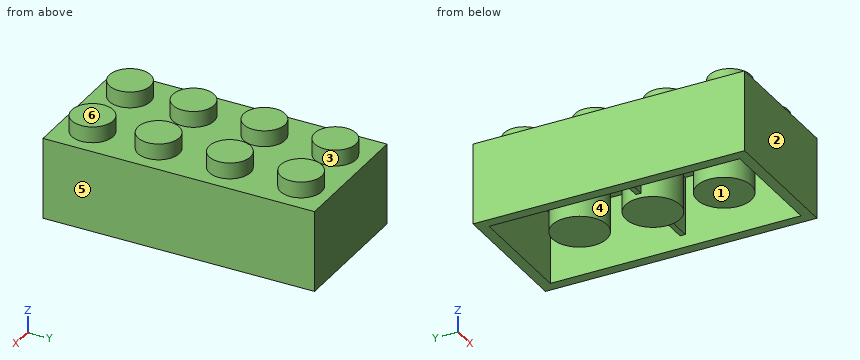
```python
from build123d import *

# Parameters (mm, degrees)
F0_W      = 15.748
F0_H      = 9.4996
F1_DEPTH  = 31.75
F2_R      = 2.413
F4_DEPTH  = 1.8796
F3_R      = 2.413
F5_DEPTH  = 1.8796
F6_T      = -1.2192
F7_R      = 3.175
F8_DEPTH  = 7.3152
F9_DEPTH  = 7.3152
F10_DEPTH = 7.3152
F12_DEPTH = 6.7881


with BuildPart() as f1:
    # F0 (on Front) → F1 (new body)
    with BuildSketch(Plane.XZ):
        with Locations((-0.199874863, 0.3277875761)):
            Rectangle(F0_W, F0_H)
    extrude(amount=F1_DEPTH)

    # F2 (on face) → F4 (join)
    with BuildSketch(Plane.XY.offset(5.0775875761)):
        with Locations((-4.2189443147, -27.9770765305)):
            Circle(F2_R)
        with Locations((3.9266556272, -27.978049837)):
            Circle(F2_R)
    extrude(amount=F4_DEPTH)

    # F3 (on face) → F5 (join)
    with BuildSketch(Plane.XY.offset(5.0775875761)):
        with Locations((3.7918896414, -20.3214651638)):
            Circle(F3_R)
        with Locations((3.75443, -12.0085638718)):
            Circle(F3_R)
        with Locations((3.7169703586, -3.6956625797)):
            Circle(F3_R)
        with Locations((-3.7169703586, -3.6956625797)):
            Circle(F3_R)
        with Locations((-3.75443, -12.0085638718)):
            Circle(F3_R)
        with Locations((-3.7918896414, -20.3214651638)):
            Circle(F3_R)
    extrude(amount=F5_DEPTH)

    # F6
    f6_openings = [f1.faces().sort_by_distance(p)[0] for p in [
        (-0.199875, -15.875, -4.422012),
    ]]
    offset(amount=F6_T, openings=f6_openings, kind=Kind.INTERSECTION)

    # F7 (on face) → F8 (join)
    with BuildSketch(Plane(origin=(0, 0, 3.8583875761), x_dir=(1, 0, 0), z_dir=(0, 0, -1))):
        with Locations((0, 8.1207330356)):
            Circle(F7_R)
    extrude(amount=F8_DEPTH)

    # F7 (on face) → F9 (join)
    with BuildSketch(Plane(origin=(0, 0, 3.8583875761), x_dir=(1, 0, 0), z_dir=(0, 0, -1))):
        with Locations((0, 25.0235652365)):
            Circle(F7_R)
    extrude(amount=F9_DEPTH)

    # F7 (on face) → F10 (join)
    with BuildSketch(Plane(origin=(0, 0, 3.8583875761), x_dir=(1, 0, 0), z_dir=(0, 0, -1))):
        with BuildLine():
            ThreePointArc((-3.175, 16.6939621039), (0, 13.5189621039), (3.175, 16.6939621039))
            ThreePointArc((3.175, 16.6939621039), (0, 19.8689621039), (-3.175, 16.6939621039))
        make_face()
    extrude(amount=F10_DEPTH)

    # F11 (on face) → F12 (join)
    with BuildSketch(Plane(origin=(0, 0, 3.8583875761), x_dir=(1, 0, 0), z_dir=(0, 0, -1))):
        with BuildLine():
            ThreePointArc((-3.1611326952, 16.3975416535), (-3.1749888394, 16.7023805357), (-3.1595163506, 17.0071416535))
            Line((-3.1595163506, 17.0071416535), (-6.854674863, 17.0071416535))
            Line((-6.854674863, 17.0071416535), (-6.854674863, 16.3975416535))
            Line((-6.854674863, 16.3975416535), (-3.1611326952, 16.3975416535))
        make_face()
        with BuildLine():
            Line((6.454925137, 17.0071416535), (3.1595163506, 17.0071416535))
            ThreePointArc((3.1595163506, 17.0071416535), (3.1711267251, 16.8507431404), (3.175, 16.6939621039))
            ThreePointArc((3.175, 16.6939621039), (3.171531279, 16.5455897804), (3.1611326952, 16.3975416535))
            Line((3.1611326952, 16.3975416535), (6.454925137, 16.3975416535))
            Line((6.454925137, 16.3975416535), (6.454925137, 17.0071416535))
        make_face()
    extrude(amount=F12_DEPTH)


solid = f1.part
```
Work out the finished part from the listing and answer in its coordinate system (mm). Face numbers are marked on the shaded views. A direction names the side the tool comes from. Coordinates: 2 decimals unless noted, no trailing zeros. Write each loop counter-clockwise with the first axis right and the second up, starting at its lowest first coordinate (ties: lowest second). Pieces come first, ordered by that corner, then holes.
Q1. Find the intervals of material crossed by line 1 (Y direction, x = 5.5, z = 2.5); line 2 (X direction, y = -8, z = 2.5); line 3 (Y direction, x = 0, z = -1), in increasing order.
Q2. Each of these flat-tipped pins is pushed along its axis until it touches: pin 1 Ø2.5 at (x, z) = (4.5, 1) entering from +Y; pin 2 Ø1.2 at (x, y) = (-5, -28) entering from -Z; pin 3 Ø1.2 at (x, y) = (-4, -12) entering from -Z; pin 4 Ø1.5 at (x, y) = (-2, -23) entering from -Z. Where does it stop, or does it pass through?
Q3. A cutting plane is placed at C-C, the plane z = 4.75. State how many separate pieces and enclosed holes the cut face has, then the cut area to 3 significant figures.
Q4. A cutting plane is placed at D-D, the plane y = -24.5. Give the vertices of the cut face in (x, z), then the cut area to 3 significant figures.
Q5. Determine the mould class of the marked faces 4, 5 and 6 for opening direction X: released by +X, released by -X, zero draft, split by the parting line, or undercut.
Q6. A cutting plane is placed at B-B, the plane x = 0. Give the vertices of the cut face in (y, z).
Q7. Which of the six approach directions +Z, -Z, +X, -X, +Y, -Y give full straight-line access (tool end or side, diameter ignored) to the marked faces 1, 2 and 3?
Q8. A cutting plane is placed at A-A, the plane z = 3.25. Give the vertices of the cut face in (x, y) (3 decimals), then the cut area to 3 significant figures.
Findings below:
1. line 1: y = -31.75 to -30.53, -17.01 to -16.4, -1.22 to 0
1. line 2: x = -8.07 to -6.85, -3.17 to 3.17, 6.45 to 7.67
1. line 3: y = -31.75 to -30.53, -28.2 to -21.85, -19.87 to -13.52, -11.3 to -4.95, -1.22 to 0
2. pin 1: stops at y = 0
2. pin 2: stops at z = 3.86
2. pin 3: stops at z = 5.74
2. pin 4: stops at z = -3.46
3. separate pieces: 1
3. enclosed holes: 8
3. area: 464 mm2
4. outline: (-8.07, -4.42) - (-6.85, -4.42) - (-6.85, 3.86) - (-3.13, 3.86) - (-3.13, -3.46) - (3.13, -3.46) - (3.13, 3.86) - (6.45, 3.86) - (6.45, -4.42) - (7.67, -4.42) - (7.67, 5.08) - (-8.07, 5.08) - close
4. area: 85.2 mm2
5. face 4: undercut
5. face 5: released by +X
5. face 6: zero draft
6. outline: (-31.75, -4.42) - (-30.53, -4.42) - (-30.53, 3.86) - (-28.2, 3.86) - (-28.2, -3.46) - (-21.85, -3.46) - (-21.85, 3.86) - (-19.87, 3.86) - (-19.87, -3.46) - (-13.52, -3.46) - (-13.52, 3.86) - (-11.3, 3.86) - (-11.3, -3.46) - (-4.95, -3.46) - (-4.95, 3.86) - (-1.22, 3.86) - (-1.22, -4.42) - (0, -4.42) - (0, 5.08) - (-31.75, 5.08) - close
7. face 1: -Z
7. face 2: +Z, -Z, +X, -X, -Y
7. face 3: +Z
8. outline: (-8.074, -31.75) - (7.674, -31.75) - (7.674, 0) - (-8.074, 0) - close; circle Ø6.35 at (0, -25.024); circle Ø6.35 at (0, -8.121); hole (-6.855, -30.531) - (6.455, -30.531) - (6.455, -17.007) - (3.16, -17.007) arc R3.175 cw to (-3.16, -17.007) - (-6.855, -17.007) - close; hole (-6.855, -16.398) - (-3.161, -16.398) arc R3.175 cw to (3.161, -16.398) - (6.455, -16.398) - (6.455, -1.219) - (-6.855, -1.219) - close
8. area: 209 mm2
